Design review of the part built by this model. Coordinates are the model's own, in mm. Face numbers are marked on the shaded views. A direction names the side the tool comes from. Coordinates: 2 decimals unless noted, no trailing zeros. Write each loop counter-clockwise with the first axis right and the second up, starting at its lowest first coordinate (ties: lowest second). Pieces come first, ordered by that corner, then holes.
```python
from build123d import *

# Parameters (mm, degrees)
MAIN_DEPTH                                   = 107.5
F_4_0MM_DOWEL_HOLE1_D                        = 4.1
F_4_0MM_DOWEL_HOLE1_ON_FACE_2_D              = 4.1
F_4_0MM_DOWEL_HOLE1_ON_FACE_3_D              = 4.1
F_4_0MM_DOWEL_HOLE1_ON_FACE_4_D              = 4.1
SKETCH4_W                                    = 10
SKETCH4_H                                    = 20
BATTERY_STRAP_CUTOUT_DEPTH                   = 150.511994765
BATTERY_STRAP_CUTOUT_MIRROR_AT_THE_S_2_W     = 10
BATTERY_STRAP_CUTOUT_MIRROR_AT_THE_S_2_H     = 20
BATTERY_STRAP_CUTOUT_MIRROR_AT_THE_S_3_DEPTH = 150.511994765
BATTERY_MOUNT_DEPTH                          = 17.5
PCB_MOUNTS_REACH                             = 152.392
SKETCH7_R                                    = 4
SKETCH8_R                                    = 2.05
PCB_MOUNT_INSERTS_DEPTH                      = 5.7
SKETCH9_R                                    = 1.6
FEET_SCREW_HOLE_DEPTH                        = 151.392275662
MIRROR1_AT_THE_SECOND_PLANE_COPY_1_SKETC_R   = 1.6
MIRROR1_AT_THE_SECOND_PLANE_COPY_1_DEPTH     = 151.392275662


with BuildPart() as part:
    # Sketch2 → Main (new, symmetric)
    with BuildSketch(Plane(origin=(0, 0, 0), x_dir=(0, 0, -1), z_dir=(1, 0, 0))):
        Polygon((-85, 0), (85, 0), (97.5, 12.5), (103.156854249, 6.843145751), (88.313708499, -8), (-88.313708499, -8), (-103.156854249, 6.843145751), (-97.5, 12.5), align=None)
    extrude(amount=MAIN_DEPTH, both=True)

    # Ø4.0mm Dowel Hole1 (through all)
    with Locations(Plane(origin=(-102.5, 7.071067812, -92.071067812), x_dir=(0, 0.707106781187, -0.707106781187), z_dir=(0, 0.707106781187, 0.707106781187))):
        with Locations((0, 0)):
            Hole(F_4_0MM_DOWEL_HOLE1_D / 2)

    # Ø4.0mm Dowel Hole1 on face 2 (through all)
    with Locations(Plane(origin=(-102.5, 0, -75), x_dir=(0, 0, 1), z_dir=(0, 1, 0))):
        with Locations((0, 0), (75, 0), (150, 0), (150, 205), (75, 205), (0, 205)):
            Hole(F_4_0MM_DOWEL_HOLE1_ON_FACE_2_D / 2)

    # Ø4.0mm Dowel Hole1 on face 3 (through all)
    with Locations(Plane(origin=(-102.5, 7.071067812, 92.071067812), x_dir=(0, -0.707106781187, -0.707106781187), z_dir=(0, 0.707106781187, -0.707106781187))):
        with Locations((0, 0), (0, -205)):
            Hole(F_4_0MM_DOWEL_HOLE1_ON_FACE_3_D / 2)

    # Ø4.0mm Dowel Hole1 on face 4 (through all)
    with Locations(Plane(origin=(102.5, 7.071067812, -92.071067812), x_dir=(0, 0.707106781187, -0.707106781187), z_dir=(0, 0.707106781187, 0.707106781187))):
        with Locations((0, 0)):
            Hole(F_4_0MM_DOWEL_HOLE1_ON_FACE_4_D / 2)

    # Sketch4 → Battery strap cutout (cut, through all)
    with BuildSketch(Plane(origin=(0, 0, 0), x_dir=(1, 0, 0), z_dir=(0, 1, 0))):
        with Locations((22.5, 52.5)):
            Rectangle(SKETCH4_W, SKETCH4_H)
    battery_strap_cutout = extrude(amount=-BATTERY_STRAP_CUTOUT_DEPTH, mode=Mode.SUBTRACT)

    # Battery strap cutout mirror: Battery strap cutout across plane
    add(battery_strap_cutout.mirror(Plane(origin=(0, 0, 0), x_dir=(0, 0, 1), z_dir=(1, 0, 0))), mode=Mode.SUBTRACT)

    # Battery strap cutout mirror at the secon: Battery strap cutout across plane
    add(battery_strap_cutout.mirror(Plane.XY), mode=Mode.SUBTRACT)

    # Battery strap cutout mirror at the s 2 → Battery strap cutout mirror at the s 3 (cut, through all)
    with BuildSketch(Plane(origin=(0, 0, 0), x_dir=(-1, 0, 0), z_dir=(0, 1, 0))):
        with Locations((22.5, 52.5)):
            Rectangle(BATTERY_STRAP_CUTOUT_MIRROR_AT_THE_S_2_W, BATTERY_STRAP_CUTOUT_MIRROR_AT_THE_S_2_H)
    extrude(amount=-BATTERY_STRAP_CUTOUT_MIRROR_AT_THE_S_3_DEPTH, mode=Mode.SUBTRACT)

    # Sketch6 → Battery mount (add, symmetric)
    with BuildSketch(Plane(origin=(0, 0, 0), x_dir=(0, 0, -1), z_dir=(1, 0, 0))):
        Polygon((-97.5, 12.5), (97.5, 12.5), (85, 0), (-85, 0), align=None)
    extrude(amount=BATTERY_MOUNT_DEPTH, both=True)

    # PCB mounts: up to this face of the body (flat: up to its plane)
    pcb_mounts_end = Plane(part.part.faces().sort_by_distance((63.47007498, 0, 0))[0])
    # Sketch7 → PCB mounts (add, up to the picked face)
    with BuildSketch(Plane(origin=(0, 12.5, 0), x_dir=(1, 0, 0), z_dir=(0, 1, 0)), mode=Mode.PRIVATE) as pcb_mounts_sk1:
        with Locations(Location((-50, -15, 0), (0, 0, 270))):
            Circle(SKETCH7_R)
    pcb_mounts_tool1 = split(extrude(pcb_mounts_sk1.sketch, amount=-PCB_MOUNTS_REACH, mode=Mode.PRIVATE), bisect_by=pcb_mounts_end, keep=Keep.BOTH, mode=Mode.PRIVATE)
    # Sketch7 → PCB mounts (add, up to the picked face)
    with BuildSketch(Plane(origin=(0, 12.5, 0), x_dir=(1, 0, 0), z_dir=(0, 1, 0)), mode=Mode.PRIVATE) as pcb_mounts_sk2:
        with Locations(Location((-50, -83, 0), (0, 0, 270))):
            Circle(SKETCH7_R)
    pcb_mounts_tool2 = split(extrude(pcb_mounts_sk2.sketch, amount=-PCB_MOUNTS_REACH, mode=Mode.PRIVATE), bisect_by=pcb_mounts_end, keep=Keep.BOTH, mode=Mode.PRIVATE)
    # Sketch7 → PCB mounts (add, up to the picked face)
    with BuildSketch(Plane(origin=(0, 12.5, 0), x_dir=(1, 0, 0), z_dir=(0, 1, 0)), mode=Mode.PRIVATE) as pcb_mounts_sk3:
        with Locations(Location((-61, -83, 0), (0, 0, 270))):
            Circle(SKETCH7_R)
    pcb_mounts_tool3 = split(extrude(pcb_mounts_sk3.sketch, amount=-PCB_MOUNTS_REACH, mode=Mode.PRIVATE), bisect_by=pcb_mounts_end, keep=Keep.BOTH, mode=Mode.PRIVATE)
    # Sketch7 → PCB mounts (add, up to the picked face)
    with BuildSketch(Plane(origin=(0, 12.5, 0), x_dir=(1, 0, 0), z_dir=(0, 1, 0)), mode=Mode.PRIVATE) as pcb_mounts_sk4:
        with Locations(Location((-50, 73, 0), (0, 0, 270))):
            Circle(SKETCH7_R)
    pcb_mounts_tool4 = split(extrude(pcb_mounts_sk4.sketch, amount=-PCB_MOUNTS_REACH, mode=Mode.PRIVATE), bisect_by=pcb_mounts_end, keep=Keep.BOTH, mode=Mode.PRIVATE)
    # Sketch7 → PCB mounts (add, up to the picked face)
    with BuildSketch(Plane(origin=(0, 12.5, 0), x_dir=(1, 0, 0), z_dir=(0, 1, 0)), mode=Mode.PRIVATE) as pcb_mounts_sk5:
        with Locations(Location((-50, 5, 0), (0, 0, 270))):
            Circle(SKETCH7_R)
    pcb_mounts_tool5 = split(extrude(pcb_mounts_sk5.sketch, amount=-PCB_MOUNTS_REACH, mode=Mode.PRIVATE), bisect_by=pcb_mounts_end, keep=Keep.BOTH, mode=Mode.PRIVATE)
    # Sketch7 → PCB mounts (add, up to the picked face)
    with BuildSketch(Plane(origin=(0, 12.5, 0), x_dir=(1, 0, 0), z_dir=(0, 1, 0)), mode=Mode.PRIVATE) as pcb_mounts_sk6:
        with Locations(Location((-61, 5, 0), (0, 0, 270))):
            Circle(SKETCH7_R)
    pcb_mounts_tool6 = split(extrude(pcb_mounts_sk6.sketch, amount=-PCB_MOUNTS_REACH, mode=Mode.PRIVATE), bisect_by=pcb_mounts_end, keep=Keep.BOTH, mode=Mode.PRIVATE)
    # Sketch7 → PCB mounts (add, up to the picked face)
    with BuildSketch(Plane(origin=(0, 12.5, 0), x_dir=(1, 0, 0), z_dir=(0, 1, 0)), mode=Mode.PRIVATE) as pcb_mounts_sk7:
        with Locations(Location((61, 83, 0), (0, 0, 270))):
            Circle(SKETCH7_R)
    pcb_mounts_tool7 = split(extrude(pcb_mounts_sk7.sketch, amount=-PCB_MOUNTS_REACH, mode=Mode.PRIVATE), bisect_by=pcb_mounts_end, keep=Keep.BOTH, mode=Mode.PRIVATE)
    # Sketch7 → PCB mounts (add, up to the picked face)
    with BuildSketch(Plane(origin=(0, 12.5, 0), x_dir=(1, 0, 0), z_dir=(0, 1, 0)), mode=Mode.PRIVATE) as pcb_mounts_sk8:
        with Locations(Location((50, 83, 0), (0, 0, 270))):
            Circle(SKETCH7_R)
    pcb_mounts_tool8 = split(extrude(pcb_mounts_sk8.sketch, amount=-PCB_MOUNTS_REACH, mode=Mode.PRIVATE), bisect_by=pcb_mounts_end, keep=Keep.BOTH, mode=Mode.PRIVATE)
    # Sketch7 → PCB mounts (add, up to the picked face)
    with BuildSketch(Plane(origin=(0, 12.5, 0), x_dir=(1, 0, 0), z_dir=(0, 1, 0)), mode=Mode.PRIVATE) as pcb_mounts_sk9:
        with Locations(Location((50, 15, 0), (0, 0, 270))):
            Circle(SKETCH7_R)
    pcb_mounts_tool9 = split(extrude(pcb_mounts_sk9.sketch, amount=-PCB_MOUNTS_REACH, mode=Mode.PRIVATE), bisect_by=pcb_mounts_end, keep=Keep.BOTH, mode=Mode.PRIVATE)
    # Sketch7 → PCB mounts (add, up to the picked face)
    with BuildSketch(Plane(origin=(0, 12.5, 0), x_dir=(1, 0, 0), z_dir=(0, 1, 0)), mode=Mode.PRIVATE) as pcb_mounts_sk10:
        with Locations(Location((61, -5, 0), (0, 0, 270))):
            Circle(SKETCH7_R)
    pcb_mounts_tool10 = split(extrude(pcb_mounts_sk10.sketch, amount=-PCB_MOUNTS_REACH, mode=Mode.PRIVATE), bisect_by=pcb_mounts_end, keep=Keep.BOTH, mode=Mode.PRIVATE)
    # Sketch7 → PCB mounts (add, up to the picked face)
    with BuildSketch(Plane(origin=(0, 12.5, 0), x_dir=(1, 0, 0), z_dir=(0, 1, 0)), mode=Mode.PRIVATE) as pcb_mounts_sk11:
        with Locations(Location((50, -5, 0), (0, 0, 270))):
            Circle(SKETCH7_R)
    pcb_mounts_tool11 = split(extrude(pcb_mounts_sk11.sketch, amount=-PCB_MOUNTS_REACH, mode=Mode.PRIVATE), bisect_by=pcb_mounts_end, keep=Keep.BOTH, mode=Mode.PRIVATE)
    # Sketch7 → PCB mounts (add, up to the picked face)
    with BuildSketch(Plane(origin=(0, 12.5, 0), x_dir=(1, 0, 0), z_dir=(0, 1, 0)), mode=Mode.PRIVATE) as pcb_mounts_sk12:
        with Locations(Location((50, -73, 0), (0, 0, 270))):
            Circle(SKETCH7_R)
    pcb_mounts_tool12 = split(extrude(pcb_mounts_sk12.sketch, amount=-PCB_MOUNTS_REACH, mode=Mode.PRIVATE), bisect_by=pcb_mounts_end, keep=Keep.BOTH, mode=Mode.PRIVATE)
    add(pcb_mounts_tool1.solids().sort_by(Axis((-50, 12.5, 15), (0, -1, 0)))[0])
    add(pcb_mounts_tool2.solids().sort_by(Axis((-50, 12.5, 83), (0, -1, 0)))[0])
    add(pcb_mounts_tool3.solids().sort_by(Axis((-61, 12.5, 83), (0, -1, 0)))[0])
    add(pcb_mounts_tool4.solids().sort_by(Axis((-50, 12.5, -73), (0, -1, 0)))[0])
    add(pcb_mounts_tool5.solids().sort_by(Axis((-50, 12.5, -5), (0, -1, 0)))[0])
    add(pcb_mounts_tool6.solids().sort_by(Axis((-61, 12.5, -5), (0, -1, 0)))[0])
    add(pcb_mounts_tool7.solids().sort_by(Axis((61, 12.5, -83), (0, -1, 0)))[0])
    add(pcb_mounts_tool8.solids().sort_by(Axis((50, 12.5, -83), (0, -1, 0)))[0])
    add(pcb_mounts_tool9.solids().sort_by(Axis((50, 12.5, -15), (0, -1, 0)))[0])
    add(pcb_mounts_tool10.solids().sort_by(Axis((61, 12.5, 5), (0, -1, 0)))[0])
    add(pcb_mounts_tool11.solids().sort_by(Axis((50, 12.5, 5), (0, -1, 0)))[0])
    add(pcb_mounts_tool12.solids().sort_by(Axis((50, 12.5, 73), (0, -1, 0)))[0])

    # Sketch8 → PCB mount inserts (cut)
    with BuildSketch(Plane(origin=(0, 12.5, 0), x_dir=(1, 0, 0), z_dir=(0, 1, 0))):
        with Locations(Location((-50, 73, 0), (0, 0, 270))):
            Circle(SKETCH8_R)
        with Locations(Location((-50, 5, 0), (0, 0, 270))):
            Circle(SKETCH8_R)
        with Locations(Location((-61, 5, 0), (0, 0, 270))):
            Circle(SKETCH8_R)
        with Locations(Location((-50, -15, 0), (0, 0, 270))):
            Circle(SKETCH8_R)
        with Locations(Location((-61, -83, 0), (0, 0, 270))):
            Circle(SKETCH8_R)
        with Locations(Location((-50, -83, 0), (0, 0, 270))):
            Circle(SKETCH8_R)
        with Locations(Location((50, -73, 0), (0, 0, 270))):
            Circle(SKETCH8_R)
        with Locations(Location((61, -5, 0), (0, 0, 270))):
            Circle(SKETCH8_R)
        with Locations(Location((50, -5, 0), (0, 0, 270))):
            Circle(SKETCH8_R)
        with Locations(Location((50, 15, 0), (0, 0, 270))):
            Circle(SKETCH8_R)
        with Locations(Location((61, 83, 0), (0, 0, 270))):
            Circle(SKETCH8_R)
        with Locations(Location((50, 83, 0), (0, 0, 270))):
            Circle(SKETCH8_R)
    extrude(amount=-PCB_MOUNT_INSERTS_DEPTH, mode=Mode.SUBTRACT)

    # Sketch9 → Feet screw hole (cut, through all)
    with BuildSketch(Plane.XZ.offset(8)):
        with Locations(Location((85, 70, 0), (0, 0, 270))):
            Circle(SKETCH9_R)
    feet_screw_hole = extrude(amount=-FEET_SCREW_HOLE_DEPTH, mode=Mode.SUBTRACT)

    # Mirror1: Feet screw hole across plane
    add(feet_screw_hole.mirror(Plane.XY), mode=Mode.SUBTRACT)

    # Mirror1 at the second plane: Feet screw hole across plane
    add(feet_screw_hole.mirror(Plane(origin=(0, 0, 0), x_dir=(0, 0, 1), z_dir=(1, 0, 0))), mode=Mode.SUBTRACT)

    # Mirror1 at the second plane copy 1 sketc → Mirror1 at the second plane copy 1 (cut, through all)
    with BuildSketch(Plane(origin=(0, -8, 0), x_dir=(-1, 0, 0), z_dir=(0, -1, 0))):
        with Locations(Location((85, 70, 0), (0, 0, 270))):
            Circle(MIRROR1_AT_THE_SECOND_PLANE_COPY_1_SKETC_R)
    extrude(amount=-MIRROR1_AT_THE_SECOND_PLANE_COPY_1_DEPTH, mode=Mode.SUBTRACT)


solid = part.part
```
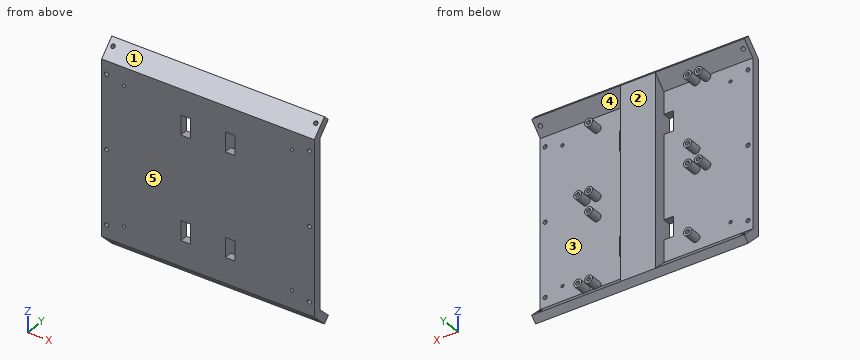
(1) Wall thickness on line 1 (X direction, y = 7.5, z = 15); line 2 (X direction, y = -2, z = -75); line 3 (X direction, y = 9.85, z = 5): over which ranges is each line inside the solid? List them lowest first.
(2) Insertion check: pin 1 Ø5 at (x, y) = (8.5, 0.5) entering from -Z; pin 2 Ø1.5 at (x, z) = (-59, -68) entering from +Y; pin 3 Ø9 at (x, y) = (-21, -5) entering from +Z. Each pin has a flat end and moves straight along its axis. Give the tip position at first contact, or say it passes through.
(3) Consider section C-C (z = -32.5). Give the boundary of the cut face in (x, y).
(4) Consider section A-A (z = 53.5). Give the boundary of the cut face in (x, y), plus the area to 3 significant figures.
(5) Consider section D-D (y = -4.25). State how many separate pieces and enclosed holes the cut face has, plus the area to 3 significant figures.
(6) Consider section B-B (x = 38). Give the boundary of the cut face in (y, z), plus the area to 3 significant figures.
(7) Mouldability with a two-part tool opening along Z and no side actions: class the marked faces 1, 2 and 3 as +Z half, -Z half, draft (parallel to the pull), parting line (faces both ways), or undercut.
(8) For the marked faces 4 and 5, list the 3-axis set-ups (+Z, -Z, +X, -X, +Y, -Y) from which the entire face can be reached by the end or side of a thin tool; tool diameter is ignored.
Results:
1. line 1: x = -54 to -52.05, -47.95 to -46, -17.5 to 17.5
1. line 2: x = -107.5 to -104.55, -100.45 to 100.45, 104.55 to 107.5
1. line 3: x = -17.5 to 17.5, 46 to 47.95, 52.05 to 54, 57 to 58.95, 63.05 to 65
2. pin 1: stops at z = -99.31
2. pin 2: stops at y = 0
2. pin 3: stops at z = 95.81
3. outline: (-107.5, -8) - (107.5, -8) - (107.5, 0) - (17.5, 0) - (17.5, 12.5) - (-17.5, 12.5) - (-17.5, 0) - (-107.5, 0) - close
4. outline: (-107.5, -8) - (-27.5, -8) - (-27.5, 0) - (-107.5, 0) - close; (-17.5, -8) - (17.5, -8) - (17.5, 12.5) - (-17.5, 12.5) - close; (27.5, -8) - (107.5, -8) - (107.5, 0) - (27.5, 0) - close
4. area: 2,000 mm2
5. separate pieces: 1
5. enclosed holes: 14
5. area: 38,700 mm2
6. outline: (-8, -88.31) - (6.84, -103.16) - (12.5, -97.5) - (0, -85) - (0, 85) - (12.5, 97.5) - (6.84, 103.16) - (-8, 88.31) - close
6. area: 1,700 mm2
7. face 1: +Z half
7. face 2: draft
7. face 3: undercut
8. face 4: +X, +Y
8. face 5: +Z, -Z, +X, -X, -Y
